Source: CAD feature listing. Evaluate the final solid. Frame: model axes, mm. Face numbers are marked on the shaded views. A direction names the side the tool comes from. Round coordinates to 2 decimals unless told otherwise and drop trailing zeros. Write each loop counter-clockwise with the first axis right and the second up, starting at its lowest first coordinate (ties: lowest second). Pieces come first, ordered by that corner, then holes. Notation, with made-up numbers: M 25.25,-24 L 55.25,-24 A27 ccw 55.25,12 Z; hole C 63.5,-21.5 d7. An arc over 180 degrees is marked long. Answer in a Markdown table with one row per item.
from build123d import *

# Parameters (mm, degrees)
SKETCH_1_R          = 3.5
EXTRUDE_1_DEPTH     = 29.5
SKETCH_3_W          = 37
SKETCH_3_H          = 17
CUT_EXTRUDE_2_DEPTH = 20
CUT_EXTRUDE_3_REACH = 60.849
SKETCH_4_W          = 37
SKETCH_4_H          = 45
SKETCH_4_W_2        = 35
SKETCH_4_H_2        = 14
HOLE_WIZARD_M4_1_D  = 4.3
CHAMFER_1_SIZE      = 7


with BuildPart() as part:
    # 草图1 → 凸台-拉伸1 (new, symmetric)
    with BuildSketch(Plane(origin=(0, 0, 0), x_dir=(0, 0, -1), z_dir=(1, 0, 0))):
        Polygon((0, 8), (0, 25), (23, 25), (23, 8), (48, 8), (48, 0), (-19, 0), (-19, 8), align=None)
        with Locations((13, 18)):
            Circle(SKETCH_1_R, mode=Mode.SUBTRACT)
    extrude(amount=EXTRUDE_1_DEPTH, both=True)

    # 草图3 → 切除-拉伸2 (cut)
    with BuildSketch(Plane(origin=(0, 0, -23), x_dir=(-1, 0, 0), z_dir=(0, 0, -1))):
        with Locations((0, 16.5)):
            Rectangle(SKETCH_3_W, SKETCH_3_H)
    extrude(amount=-CUT_EXTRUDE_2_DEPTH, mode=Mode.SUBTRACT)

    # 草图4 → 切除-拉伸3 (cut, up to next)
    with BuildSketch(Plane(origin=(0, 8, 0), x_dir=(1, 0, 0), z_dir=(0, 1, 0)), mode=Mode.PRIVATE) as cut_extrude_3_sk1:
        with Locations((0, 25.5)):
            Rectangle(SKETCH_4_W, SKETCH_4_H)
    cut_extrude_3_tool1 = extrude(cut_extrude_3_sk1.sketch, amount=-CUT_EXTRUDE_3_REACH, mode=Mode.PRIVATE) & part.part
    # 草图4 → 切除-拉伸3 (cut, up to next)
    with BuildSketch(Plane(origin=(0, 8, 0), x_dir=(1, 0, 0), z_dir=(0, 1, 0)), mode=Mode.PRIVATE) as cut_extrude_3_sk2:
        with Locations((0, -12)):
            Rectangle(SKETCH_4_W_2, SKETCH_4_H_2)
    cut_extrude_3_tool2 = extrude(cut_extrude_3_sk2.sketch, amount=-CUT_EXTRUDE_3_REACH, mode=Mode.PRIVATE) & part.part
    add(cut_extrude_3_tool1.solids().sort_by_distance((0, 8, -25.5))[0], mode=Mode.SUBTRACT)
    add(cut_extrude_3_tool2.solids().sort_by_distance((0, 8, 12))[0], mode=Mode.SUBTRACT)

    # M4 间隙孔1 (through all)
    with Locations(Plane(origin=(0, 0, 0), x_dir=(-1, 0, 0), z_dir=(0, -1, 0))):
        with Locations((24, -14), (24, 43), (-24, -14), (-24, 43)):
            Hole(HOLE_WIZARD_M4_1_D / 2)

    # 倒角1
    # the kernel refuses this chamfer: 7 mm, written as the material it adds along each edge
    with BuildSketch(Plane(origin=(-29.5, 8, 0), x_dir=(0, 0.9996219169112968, -0.027495876610586365), z_dir=(1, 0, 0))) as chamfer_1_piece_1_section:
        Polygon((CHAMFER_1_SIZE * 0.999621916911, CHAMFER_1_SIZE * 0.0274958766106), (-CHAMFER_1_SIZE * 0.0274958766106, CHAMFER_1_SIZE * 0.999621916911), (0, 0), align=None)
    chamfer_1_piece_1 = extrude(amount=59, mode=Mode.PRIVATE)
    chamfer_1_piece_1 = split(chamfer_1_piece_1, bisect_by=Plane(origin=(-17.5, 10.498239804, 1.946316209), z_dir=(-1, 0, 0)), keep=Keep.TOP, mode=Mode.PRIVATE)
    chamfer_1_piece_1 = split(chamfer_1_piece_1, bisect_by=Plane(origin=(-23.5, 10.498239804, 5), z_dir=(0, 0, -1)), keep=Keep.TOP, mode=Mode.PRIVATE)
    add(chamfer_1_piece_1)
    with BuildSketch(Plane(origin=(-29.5, 8, 0), x_dir=(0, 0.9996219169112968, -0.027495876610586365), z_dir=(1, 0, 0))) as chamfer_1_piece_2_section:
        Polygon((CHAMFER_1_SIZE * 0.999621916911, CHAMFER_1_SIZE * 0.0274958766106), (-CHAMFER_1_SIZE * 0.0274958766106, CHAMFER_1_SIZE * 0.999621916911), (0, 0), align=None)
    chamfer_1_piece_2 = extrude(amount=59, mode=Mode.PRIVATE)
    chamfer_1_piece_2 = split(chamfer_1_piece_2, bisect_by=Plane(origin=(-17.5, 8.493423537, 5.774901665), z_dir=(-1, 0, 0)), keep=Keep.TOP, mode=Mode.PRIVATE)
    chamfer_1_piece_2 = split(chamfer_1_piece_2, bisect_by=Plane(origin=(-23.5, 8.493423537, 5), z_dir=(0, 0, 1)), keep=Keep.TOP, mode=Mode.PRIVATE)
    add(chamfer_1_piece_2)
    with BuildSketch(Plane(origin=(-29.5, 8, 0), x_dir=(0, 0.9996219169112968, -0.027495876610586365), z_dir=(1, 0, 0))) as chamfer_1_piece_3_section:
        Polygon((CHAMFER_1_SIZE * 0.999621916911, CHAMFER_1_SIZE * 0.0274958766106), (-CHAMFER_1_SIZE * 0.0274958766106, CHAMFER_1_SIZE * 0.999621916911), (0, 0), align=None)
    chamfer_1_piece_3 = extrude(amount=59, mode=Mode.PRIVATE)
    chamfer_1_piece_3 = split(chamfer_1_piece_3, bisect_by=Plane(origin=(-17.5, 10.498239804, 1.946316209), z_dir=(1, 0, 0)), keep=Keep.TOP, mode=Mode.PRIVATE)
    chamfer_1_piece_3 = split(chamfer_1_piece_3, bisect_by=Plane(origin=(0, 10.498239804, 5), z_dir=(0, 0, -1)), keep=Keep.TOP, mode=Mode.PRIVATE)
    chamfer_1_piece_3 = split(chamfer_1_piece_3, bisect_by=Plane(origin=(17.5, 10.498239804, 1.946316209), z_dir=(-1, 0, 0)), keep=Keep.TOP, mode=Mode.PRIVATE)
    add(chamfer_1_piece_3)
    with BuildSketch(Plane(origin=(-29.5, 8, 0), x_dir=(0, 0.9996219169112968, -0.027495876610586365), z_dir=(1, 0, 0))) as chamfer_1_piece_4_section:
        Polygon((CHAMFER_1_SIZE * 0.999621916911, CHAMFER_1_SIZE * 0.0274958766106), (-CHAMFER_1_SIZE * 0.0274958766106, CHAMFER_1_SIZE * 0.999621916911), (0, 0), align=None)
    chamfer_1_piece_4 = extrude(amount=59, mode=Mode.PRIVATE)
    chamfer_1_piece_4 = split(chamfer_1_piece_4, bisect_by=Plane(origin=(23.5, 10.498239804, 5), z_dir=(0, 0, -1)), keep=Keep.TOP, mode=Mode.PRIVATE)
    chamfer_1_piece_4 = split(chamfer_1_piece_4, bisect_by=Plane(origin=(17.5, 10.498239804, 1.946316209), z_dir=(1, 0, 0)), keep=Keep.TOP, mode=Mode.PRIVATE)
    add(chamfer_1_piece_4)
    with BuildSketch(Plane(origin=(-29.5, 8, 0), x_dir=(0, 0.9996219169112968, -0.027495876610586365), z_dir=(1, 0, 0))) as chamfer_1_piece_5_section:
        Polygon((CHAMFER_1_SIZE * 0.999621916911, CHAMFER_1_SIZE * 0.0274958766106), (-CHAMFER_1_SIZE * 0.0274958766106, CHAMFER_1_SIZE * 0.999621916911), (0, 0), align=None)
    chamfer_1_piece_5 = extrude(amount=59, mode=Mode.PRIVATE)
    chamfer_1_piece_5 = split(chamfer_1_piece_5, bisect_by=Plane(origin=(23.5, 8.493423537, 5), z_dir=(0, 0, 1)), keep=Keep.TOP, mode=Mode.PRIVATE)
    chamfer_1_piece_5 = split(chamfer_1_piece_5, bisect_by=Plane(origin=(17.5, 8.493423537, 5.774901665), z_dir=(1, 0, 0)), keep=Keep.TOP, mode=Mode.PRIVATE)
    add(chamfer_1_piece_5)
    with BuildSketch(Plane(origin=(29.5, 8, -23), x_dir=(0, 0.9996219169112968, 0.02749587661058661), z_dir=(-1, 0, 0)), Plane(origin=(-18.5, 8, -23), x_dir=(0, 0.9996219169112968, 0.02749587661058661), z_dir=(-1, 0, 0))) as chamfer_1_piece_6:
        Polygon((CHAMFER_1_SIZE * 0.999621916911, CHAMFER_1_SIZE * 0.0274958766106), (-CHAMFER_1_SIZE * 0.0274958766106, CHAMFER_1_SIZE * 0.999621916911), (0, 0), align=None)
    extrude(amount=11)


solid = part.part
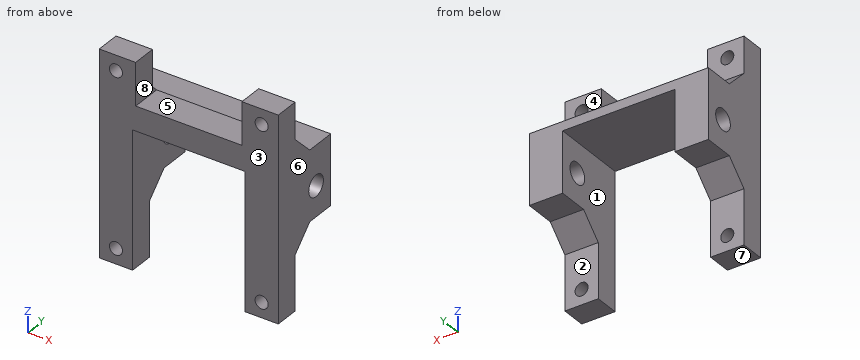
Q1. Pull-direction query (X, two-part tool) for the marked faces 6, 7 and 8; classes: pulls with the +X half, pulls with the -X half, needs draft (parallel to the pull), parting line crosses it, or undercut.
Solutions:
| item | result |
|---|---|
| face 6 | pulls with the +X half |
| face 7 | needs draft |
| face 8 | undercut |
Q2. Access query for the marked faces 1, 2, 3, 4 and 5. Directions: +Z, -Z, +X, -X, +Y, -Y. A direction counts if a zero-diameter tool reaches every point of the face in a straight line with its end or side. Return the directions, or none.
Solutions:
| item | result |
|---|---|
| face 1 | -Z, +Y, -Y |
| face 2 | -Z, +X, -X, +Y |
| face 3 | +Z, -Z, +X, -X, -Y |
| face 4 | +Z, +X, -X, +Y |
| face 5 | +Z, +Y, -Y |
Q3. Section B-B (z = -43). Return loops of the section in (x, y), and give its area (3 significant figures).
Solutions:
| item | result |
|---|---|
| outline | M -29.5,0 L -26.15,0 L -26.15,8 L -29.5,8 Z; M -21.85,0 L -18.5,0 L -18.5,8 L -21.85,8 Z; M 18.5,0 L 21.85,0 L 21.85,8 L 18.5,8 Z; M 26.15,0 L 29.5,0 L 29.5,8 L 26.15,8 Z |
| area | 107 mm2 |
Q4. Section D-D (y = 7). Return loops of the section in (x, z).
Solutions:
| item | result |
|---|---|
| outline | M -29.5,-48 L -18.5,-48 L -18.5,-3 L 18.5,-3 L 18.5,-48 L 29.5,-48 L 29.5,19 L 17.5,19 L 17.5,5 L -17.5,5 L -17.5,19 L -29.5,19 Z; hole C -24,-43 d4.3; hole C -24,14 d4.3; hole C 24,-43 d4.3; hole C 24,14 d4.3 |
Q5. Contact query for flat-ended pins moving along their axis: pin 1 Ø5 at (x, y) = (26, 22) entering from -Z; pin 2 Ø5 at (x, z) = (24, 14) entering from +Y; pin 3 Ø5 at (x, y) = (-5.5, 4) entering from +Z; pin 4 Ø2.5 at (x, z) = (-24, 14) entering from +Y. Output: stop coordinate, or through.
Solutions:
| item | result |
|---|---|
| pin 1 | stops at z = -23 |
| pin 2 | stops at y = 8 |
| pin 3 | stops at z = 5 |
| pin 4 | passes through |
Q6. Section A-A (y = 18). Return loops of the section in (x, z), and give its area (3 significant figures).
Solutions:
| item | result |
|---|---|
| outline | M -29.5,-23 L -18.5,-23 L -18.5,-16.5 L -29.5,-16.5 Z; M -29.5,-9.5 L -18.5,-9.5 L -18.5,-3 L 18.5,-3 L 18.5,-9.5 L 29.5,-9.5 L 29.5,0 L -29.5,0 Z; M 18.5,-23 L 29.5,-23 L 29.5,-16.5 L 18.5,-16.5 Z |
| area | 463 mm2 |
Q7. Section C-C (x = 24). Return loops of the section in (y, z).
Solutions:
| item | result |
|---|---|
| outline | M 0,-48 L 8,-48 L 8,-45.15 L 0,-45.15 Z; M 0,-40.85 L 8,-40.85 L 8,-30 L 15,-23 L 25,-23 L 25,0 L 15,0 L 8,7 L 8,11.85 L 0,11.85 Z; M 0,16.15 L 8,16.15 L 8,19 L 0,19 Z; hole C 18,-13 d7 |
Q8. Material intervals for probe 1 along X at (y, z) = (3.75, -43); probe 2 along X at (y, z) = (6.75, 14); probe 3 along Z at (x, y) = (24, 4), sorted ascending.
Solutions:
| item | result |
|---|---|
| probe 1 | x = -29.5 to -26.15, -21.85 to -18.5, 18.5 to 21.85, 26.15 to 29.5 |
| probe 2 | x = -29.5 to -26.15, -21.85 to -17.5, 17.5 to 21.85, 26.15 to 29.5 |
| probe 3 | z = -48 to -45.15, -40.85 to 11.85, 16.15 to 19 |
